Build history of the part. All positions in model axes, mm. A direction names the side the tool comes from. Round coordinates to 2 decimals unless told otherwise and drop trailing zeros. Order: outer loops, then holes, each group sorted by start corner. A loop starts at its lowest first (then second) coordinate and runs counter-clockwise, first axis right, second up. Notation, with made-up numbers: M 52,-29.5 L 65,-29.5 A6 cw 65,-23.5 Z; hole C -24.75,34.25 d8. An arc over 180 degrees is marked long. One line per item, written item: value. Start each with the question number.
Item 1: Band-saw the part on B-B, the plane x = -26. Write the cut outline in (y, z).
Item 2: Two-plate mould, pull along X, no slides. Class faces 1 (the flat face through (-0.3, -18, 0.6)), 2 (the cylindrical face through (-27.39, -13.39, 0.51)), 3 (the flat face through (53, 0, 6)): +X half, -X half, draft (parallel to the pull), parting line (faces both ways), or undercut.
Item 3: Band-saw the part on D-D, the plane y = 7. Write the cut outline in (x, z).
Item 4: Band-saw the part on A-A, the plane y = -12.5. Write the cut outline in (x, z), then the cut area to 3 significant figures.
Item 5: Band-saw the part on C-C, the plane z = 6.25. Write the cut outline in (x, y), then the cut area to 3 significant figures.
Item 6: Probe L1, parallel to Y at x = -46, z = 0.8; L2, parallel to X at y = -12.5, z = 0.5; L3, parallel to X at y = -3, z = 8.5. List the from-to ranges inside material, lowest first.
Item 7: Tool access for faces 4 (the flat face through (-0.3, 18, 0.6)), 5 (the flat face through (-1, 0, 1)): list every direction of +Z, -Z, +X, -X, +Y, -Y with a clear straight run to the whole face (end or side of a thin tool).
Item 8: Pin check, flat tips, straight feed: pin 1 (3 mm diameter, centred on x = 18, y = 0.5, fed in from +Z); pin 2 (4 mm diameter, centred on y = -4.5, z = 9.5, fed in from -X). Stop position of each tip, or through.
```python
from build123d import *

# Parameters (mm, degrees)
SKETCH_1_W                  = 108
SKETCH_1_H                  = 36
EXTRUDE_1_DEPTH             = 1
HOLE_WIZARD_M4_1_AT_2_COUNT = 2
HOLE_WIZARD_M4_1_AT_2_PITCH = 20
SKETCH_4_W                  = 1
SKETCH_4_H                  = 36
EXTRUDE_2_DEPTH             = 10


with BuildPart() as part:
    # 草图1 → 凸台-拉伸1 (new body)
    with BuildSketch(Plane.XY):
        Rectangle(SKETCH_1_W, SKETCH_1_H)
    extrude(amount=EXTRUDE_1_DEPTH)

    # 草图3 → M4 螺纹孔的螺纹孔钻头1 (revolve, cut)
    with BuildSketch(Plane(origin=(-46, -12.5, 1), x_dir=(0, -1, 0), z_dir=(1, 0, 0))):
        Polygon((0, 0), (0, 10.991420021), (1.65, 10), (1.65, 0), align=None)
    hole_wizard_m4_1 = revolve(axis=Axis((-46, -12.5, 7.35), (0, 0, -1)), mode=Mode.SUBTRACT)

    # M4 螺纹孔的螺纹孔钻头1 at 2: M4 螺纹孔的螺纹孔钻头1 ×2
    with Locations(*[(i * HOLE_WIZARD_M4_1_AT_2_PITCH, 0, 0) for i in range(1, HOLE_WIZARD_M4_1_AT_2_COUNT)]):
        add(hole_wizard_m4_1, mode=Mode.SUBTRACT)

    # 镜向1: M4 螺纹孔的螺纹孔钻头1 across plane
    add(hole_wizard_m4_1.mirror(Plane.ZX), mode=Mode.SUBTRACT)

    # 镜向1 copy 1 sketch → 镜向1 copy 1 (revolve, cut)
    with BuildSketch(Plane(origin=(-26, 12.5, 1), x_dir=(0, 1, 0), z_dir=(1, 0, 0))):
        Polygon((0, 0), (0, -10.991420021), (1.65, -10), (1.65, 0), align=None)
    revolve(axis=Axis((-26, 12.5, 7.35), (0, 0, 1)), mode=Mode.SUBTRACT)

    # 草图4 → 凸台-拉伸2 (add)
    with BuildSketch(Plane.XY.offset(1)):
        with Locations((53.5, 0)):
            Rectangle(SKETCH_4_W, SKETCH_4_H)
    extrude(amount=EXTRUDE_2_DEPTH)


solid = part.part
```
Output:
1. outline: M -18,0 L -14.15,0 L -14.15,1 L -18,1 Z; M -10.85,0 L 10.85,0 L 10.85,1 L -10.85,1 Z; M 14.15,0 L 18,0 L 18,1 L 14.15,1 Z
2. face 1: draft
2. face 2: undercut
2. face 3: -X half
3. outline: M -54,0 L 54,0 L 54,11 L 53,11 L 53,1 L -54,1 Z
4. outline: M -54,0 L -47.65,0 L -47.65,1 L -54,1 Z; M -44.35,0 L -27.65,0 L -27.65,1 L -44.35,1 Z; M -24.35,0 L 54,0 L 54,11 L 53,11 L 53,1 L -24.35,1 Z
4. area: 111 mm²
5. outline: M 53,-18 L 54,-18 L 54,18 L 53,18 Z
5. area: 36.0 mm²
6. L1: y = -18 to -14.15, -10.85 to 10.85, 14.15 to 18
6. L2: x = -54 to -47.65, -44.35 to -27.65, -24.35 to 54
6. L3: x = 53 to 54
7. face 4: +Z, -Z, +X, -X, +Y
7. face 5: +Z, -X, +Y, -Y
8. pin 1: stops at z = 1
8. pin 2: stops at x = 53
